```python
from build123d import *

# Parameters (mm, degrees)
SM_BASE_FLANGE_1_DEPTH = 3
SKETCH_4_W             = 20
SKETCH_4_H             = 3
EXTRUDE_1_DEPTH        = 2
SKETCH_5_R             = 3
CUT_EXTRUDE_1_DEPTH    = 10


# Sheet-metal steps are written as plain solids
with BuildPart() as part:
    # Sketch 1 → Базовая кромка1 (new body)
    with BuildSketch(Plane.XY):
        with BuildLine():
            Line((-52.715343227, 26.180564784), (441.084656773, 26.180564784))
            ThreePointArc((441.084656773, 26.180564784), (441.862474232, 25.858382243), (442.184656773, 25.080564784))
            Line((442.184656773, 25.080564784), (442.184656773, 1.180564784))
            Line((442.184656773, 1.180564784), (-53.815343227, 1.180564784))
            Line((-53.815343227, 1.180564784), (-53.815343227, 25.080564784))
            ThreePointArc((-53.815343227, 25.080564784), (-53.493160687, 25.858382243), (-52.715343227, 26.180564784))
        make_face()
    extrude(amount=-SM_BASE_FLANGE_1_DEPTH)

    # Эскиз4 → Бобышка-Вытянуть1 (add)
    with BuildSketch(Plane(origin=(0, 26.180564784, 0), x_dir=(1, 0, 0), z_dir=(0, 1, 0))):
        with Locations((54.184656773, 1.5)):
            Rectangle(SKETCH_4_W, SKETCH_4_H)
        with Locations((334.184656773, 1.5)):
            Rectangle(SKETCH_4_W, SKETCH_4_H)
    extrude(amount=EXTRUDE_1_DEPTH)

    # Эскиз5 → Вырез-Вытянуть1 (cut)
    with BuildSketch(Plane(origin=(0, 0, -3), x_dir=(-1, 0, 0), z_dir=(0, 0, -1))):
        with Locations((-422.184656773, 13.130564784)):
            Circle(SKETCH_5_R)
        with Locations((-194.184656773, 13.130564784)):
            Circle(SKETCH_5_R)
        with Locations((33.815343227, 13.130564784)):
            Circle(SKETCH_5_R)
    extrude(amount=-CUT_EXTRUDE_1_DEPTH, mode=Mode.SUBTRACT)


solid = part.part
```
Verification items for the finished model (mm, model axes). Give positions to 0.01 mm unless a question says otherwise; leave off trailing zeros. Order: outer loops, then holes, each group sorted by start corner. A loop starts at its lowest first (then second) coordinate and runs counter-clockwise, first axis right, second up. Notation, with made-up numbers: M 56,52.25 L 105,52.25 A22 ccw 105,63.25 Z; hole C 6.25,8 d5. An arc over 180 degrees is marked long. Answer in a Markdown table with one row per item. Add a question column.
Item 1: Scan lines: probe 1 along X at (y, z) = (12.25, -0.1); probe 2 along X at (y, z) = (26.5, -0.45); probe 3 along X at (y, z) = (15.5, -1). Record each from-to range of solid material in increasing order. Write a range as from..to.
Item 2: Gauge pin test, flat ends, axial feed: pin 1 (1 mm diameter, centred on y = 27.5, z = -1.5, fed in from -X); pin 2 (1.6 mm diameter, centred on y = 27.5, z = -1.5, fed in from +X); pin 3 (1.5 mm diameter, centred on x = 410.5, z = -2, fed in from +Y). Record the tip position at first contact, or that the pin passes through.
Item 3: Section check A-A, the plane z = -2.1. Enter the section's corners in (x, y), and give its area (3 significant figures).
Item 4: Section check B-B, the plane x = 141.5. Enter the section's corners in (y, z).
Filled sheet:
| question | item | result |
|---|---|---|
| 1 | probe 1 | x = -53.82..-36.68, -30.95..191.32, 197.05..419.32, 425.05..442.18 |
| 1 | probe 2 | x = 44.18..64.18, 324.18..344.18 |
| 1 | probe 3 | x = -53.82..-35.66, -31.98..192.34, 196.02..420.34, 424.02..442.18 |
| 2 | pin 1 | stops at x = 44.18 |
| 2 | pin 2 | stops at x = 344.18 |
| 2 | pin 3 | stops at y = 26.18 |
| 3 | outline | M -53.82,1.18 L 442.18,1.18 L 442.18,25.08 A1.1 ccw 441.08,26.18 L 344.18,26.18 L 344.18,28.18 L 324.18,28.18 L 324.18,26.18 L 64.18,26.18 L 64.18,28.18 L 44.18,28.18 L 44.18,26.18 L -52.72,26.18 A1.1 ccw -53.82,25.08 Z; hole C -33.82,13.13 d6; hole C 194.18,13.13 d6; hole C 422.18,13.13 d6 |
| 3 | area | 12,400 mm^2 |
| 4 | outline | M 1.18,-3 L 26.18,-3 L 26.18,0 L 1.18,0 Z |
